Verification items for the finished model (mm, model axes). Face numbers are marked on the shaded views. Coordinates: 2 decimals unless noted, no trailing zeros. Write each loop counter-clockwise with the first axis right and the second up, starting at its lowest first coordinate (ties: lowest second). Pieces come first, ordered by that corner, then holes. Notation, with made-up numbers: (-30, 54.5) -> (-3, 54.5) arc R24 cw to (-3, 73.5) -> close; hole circle Ø9 at (71, 62.25). An arc over 180 degrees is marked (long way). Use CSV: the item, a comma, the result in double quotes.
```python
from build123d import *

# Parameters (mm, degrees)
SKETCH1_W                       = 8.390953786
SKETCH1_H                       = 32.6942
SKETCH1_H_2                     = 13
SKETCH1_H_3                     = 2.6
BOSS_EXTRUDE1_DEPTH             = 5
CUT_EXTRUDE1_DEPTH              = 51.767483063
CUT_EXTRUDE1_DEPTH_BACK         = 51.767483063
SKETCH3_W                       = 5.5
SKETCH3_H                       = 5.5
SKETCH3_R                       = 1.375
EXTRUDE_BOTTOM_SCREW_PADS_DEPTH = 1.5
SKETCH4_R                       = 2.25
CUT_BOTTOM_COUNTERSINK_DEPTH    = 0.5
SKETCH5_W                       = 5.5
SKETCH5_H                       = 5.5
SKETCH5_R                       = 1.375
EXTRUDE_SIDE_SCREW_PADS_DEPTH   = 1.5
SKETCH6_R                       = 2.25
CUT_SIDE_COUNTERSINK_DEPTH      = 0.5
FILLET_SCREW_PADS_R             = 2.25
FILLET4_R                       = 3.5
FILLET5_R                       = 0.5
SKETCH7_W                       = 13.890953786
SKETCH7_H                       = 10.5
CUT_EXTRUDE4_DEPTH              = 0.51


with BuildPart() as part:
    # Sketch1 → Boss-Extrude1 (new body)
    with BuildSketch(Plane.XZ.offset(-14.914945084)):
        with Locations((0.553417297, 5.002763775)):
            Rectangle(SKETCH1_W, SKETCH1_H)
        with Locations((0.553417297, 27.849863775)):
            Rectangle(SKETCH1_W, SKETCH1_H_2)
        with Locations((0.553417297, 35.649863775)):
            Rectangle(SKETCH1_W, SKETCH1_H_3)
    extrude(amount=BOSS_EXTRUDE1_DEPTH)

    # Sketch2 → Cut-Extrude1 (cut, two sides: drawn at the far end of the back side and taken through both)
    with BuildSketch(Plane(origin=(0, 0, -11.344336225), x_dir=(-1, 0, 0), z_dir=(0, 0, -1)).offset(-CUT_EXTRUDE1_DEPTH_BACK)):
        with BuildLine():
            Line((-2.553417297, 12.914945084), (-2.553417297, 14.914945084))
            Line((-2.553417297, 14.914945084), (1.446582703, 14.914945084))
            Line((1.446582703, 14.914945084), (1.446582703, 12.914945084))
            ThreePointArc((1.446582703, 12.914945084), (-0.553417297, 10.914945084), (-2.553417297, 12.914945084))
        make_face()
    extrude(amount=CUT_EXTRUDE1_DEPTH + CUT_EXTRUDE1_DEPTH_BACK, mode=Mode.SUBTRACT)

    # Sketch3 → Extrude Bottom Screw Pads (add)
    # profile 1 of 2: a face of its own
    with BuildSketch(Plane(origin=(0, 14.914945084, 0), x_dir=(1, 0, 0), z_dir=(0, 1, 0))):
        with Locations((7.49889419, 8.594336225)):
            Rectangle(SKETCH3_W, SKETCH3_H)
        with Locations(Location((7.49889419, 8.594336225, 0), (0, 0, 180))):
            Circle(SKETCH3_R, mode=Mode.SUBTRACT)
    # profile 2 of 2: a face of its own
    with BuildSketch(Plane(origin=(0, 14.914945084, 0), x_dir=(1, 0, 0), z_dir=(0, 1, 0))):
        with Locations((7.49889419, -34.199863775)):
            Rectangle(SKETCH3_W, SKETCH3_H)
        with Locations(Location((7.49889419, -34.199863775, 0), (0, 0, 180))):
            Circle(SKETCH3_R, mode=Mode.SUBTRACT)
    extrude(amount=-EXTRUDE_BOTTOM_SCREW_PADS_DEPTH)

    # Sketch4 → Cut Bottom Countersink (cut)
    with BuildSketch(Plane.XZ.offset(-13.414945084)):
        with Locations((7.49889419, 34.199863775)):
            Circle(SKETCH4_R)
        with Locations((7.49889419, -8.594336225)):
            Circle(SKETCH4_R)
    extrude(amount=-CUT_BOTTOM_COUNTERSINK_DEPTH, mode=Mode.SUBTRACT)

    # Sketch5 → Extrude Side Screw Pads (add)
    # profile 1 of 2: a face of its own
    with BuildSketch(Plane.ZY.offset(3.642059596)):
        with Locations((-8.594336225, 7.164945084)):
            Rectangle(SKETCH5_W, SKETCH5_H)
        with Locations(Location((-8.594336225, 7.164945084, 0), (0, 0, 270))):
            Circle(SKETCH5_R, mode=Mode.SUBTRACT)
    # profile 2 of 2: a face of its own
    with BuildSketch(Plane.ZY.offset(3.642059596)):
        with Locations((34.199863775, 7.164945084)):
            Rectangle(SKETCH5_W, SKETCH5_H)
        with Locations(Location((34.199863775, 7.164945084, 0), (0, 0, 270))):
            Circle(SKETCH5_R, mode=Mode.SUBTRACT)
    extrude(amount=-EXTRUDE_SIDE_SCREW_PADS_DEPTH)

    # Sketch6 → Cut Side Countersink (cut)
    with BuildSketch(Plane(origin=(-2.142059596, 0, 0), x_dir=(0, 0, -1), z_dir=(1, 0, 0))):
        with Locations(Location((-34.199863775, 7.164945084, 0), (0, 0, 90))):
            Circle(SKETCH6_R)
        with Locations(Location((8.594336225, 7.164945084, 0), (0, 0, 90))):
            Circle(SKETCH6_R)
    extrude(amount=-CUT_SIDE_COUNTERSINK_DEPTH, mode=Mode.SUBTRACT)

    # Fillet Screw Pads
    fillet_screw_pads_edges = [part.edges().sort_by_distance(p)[0] for p in [
        (-2.892059596, 4.414945084, 36.949863775),
        (-2.892059596, 4.414945084, 31.449863775),
        (10.24889419, 14.164945084, -11.344336225),
        (10.24889419, 14.164945084, -5.844336225),
        (10.24889419, 14.164945084, 31.449863775),
        (10.24889419, 14.164945084, 36.949863775),
        (-2.892059596, 4.414945084, -5.844336225),
        (-2.892059596, 4.414945084, -11.344336225),
    ]]
    fillet(fillet_screw_pads_edges, radius=FILLET_SCREW_PADS_R)

    # Fillet4
    fillet4_edges = [part.edges().sort_by_distance(p)[0] for p in [
        (4.74889419, 9.914945084, 12.802763775),
    ]]
    fillet(fillet4_edges, radius=FILLET4_R)

    # Fillet5
    fillet5_edges = [part.edges().sort_by_distance(p)[0] for p in [
        (2.553417297, 14.914945084, 12.802763775),
        (-1.446582703, 14.914945084, 12.802763775),
    ]]
    fillet(fillet5_edges, radius=FILLET5_R)

    # Sketch7 → Cut-Extrude4 (cut)
    with BuildSketch(Plane.XY.offset(36.949863775)):
        with Locations((3.303417297, 9.664945084)):
            Rectangle(SKETCH7_W, SKETCH7_H)
    extrude(amount=-CUT_EXTRUDE4_DEPTH, mode=Mode.SUBTRACT)


solid = part.part
```
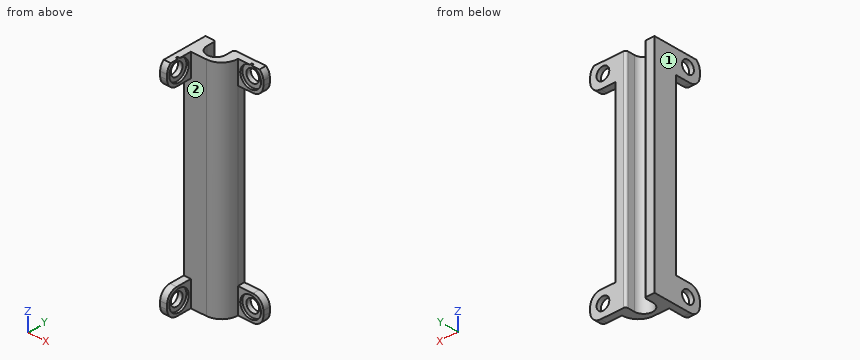
1) Cross-section at D-D (x = -0.75). Record the boundary of the cut face in (y, z), plus the area to 3 significant figures.
Return value:
outline,"(9.91, -11.34) -> (11.4, -11.34) -> (11.4, 36.44) -> (9.91, 36.44) -> close"
area,"70.9 mm2"
2) Cross-section at C-C (y = 9). Record the boundary of the cut face in (x, z), plus the area to 3 significant figures.
Return value:
outline,"(-3.64, -11.34) -> (-2.14, -11.34) -> (-2.14, -9.9) -> (-2.64, -9.9) -> (-2.64, -7.29) -> (-2.14, -7.29) -> (-2.14, -5.84) -> (-3.64, -5.84) -> close; (-3.64, 31.45) -> (-2.14, 31.45) -> (-2.14, 32.9) -> (-2.64, 32.9) -> (-2.64, 35.5) -> (-2.14, 35.5) -> (-2.14, 36.44) -> (-3.64, 36.44) -> close"
area,"13.1 mm2"
3) Mould release check, pull along Z, two halves, no side actions. Record for the marked faces 1 and 2: released by +Z, released by -Z, zero draft, split by the parting line, or undercut.
Return value:
face 1,"zero draft"
face 2,"undercut"
4) Cross-section at B-B (z = -2). Record the boundary of the cut face in (x, y).
Return value:
outline,"(-3.64, 9.91) -> (1.25, 9.91) arc R3.5 ccw to (4.75, 13.41) -> (4.75, 14.91) -> (3.05, 14.91) arc R0.5 ccw to (2.55, 14.41) -> (2.55, 12.91) arc R2 cw to (-1.45, 12.91) -> (-1.45, 14.41) arc R0.5 ccw to (-1.95, 14.91) -> (-3.64, 14.91) -> close"
5) Cross-section at A-A (y = 12.25). Record the boundary of the cut face in (x, z), plus the area to 3 significant figures.
Return value:
outline,"(-3.64, -11.34) -> (-1.33, -11.34) -> (-1.33, 36.44) -> (-3.64, 36.44) -> close; (2.44, -11.34) -> (4.55, -11.34) -> (4.55, 36.44) -> (2.44, 36.44) -> close"
area,"211 mm2"
6) Gauge pin test, flat ends, axial feed: pin 1 (6 mm diameter, centred on x = 8.5, z = -8.5, fed in from -Y); pin 2 (3.5 mm diameter, centred on y = 7.16, z = 34.2, fed in from +X); pin 3 (4 mm diameter, centred on y = 6.5, z = 33.5, fed in from +X). Record the tip position at first contact, or that the pin passes through.
Return value:
pin 1,"y = 13.41"
pin 2,"x = -2.64"
pin 3,"x = -2.14"
7) Scan lines: L1, parallel to Z at x = 8.5, y = 14.25; L2, parallel to Z at x = -2.25, y = 8; L3, parallel to X at y = 13.75, z = 1.5. Record each from-to range of solid material in increasing order.
Return value:
L1,"-11.29 to -9.54, -7.65 to -5.9, 31.51 to 33.26, 35.14 to 36.44"
L2,"-11.34 to -10.68, -6.51 to -5.84, 31.45 to 32.11, 36.29 to 36.44"
L3,"-3.64 to -1.45, 2.55 to 4.75"
